Verification items for the finished model (mm, model axes). Coordinates: 2 decimals unless noted, no trailing zeros. Loops run counter-clockwise (first coordinate to the right, second up) from the corner with the lowest first, then second, coordinate; pieces in that order, holes last. Notation, with made-up numbers: (64, -34) - (118, -34) arc R16 cw to (118, -4) - close; hole circle Ø9 at (-1.75, 58.25). An arc over 180 degrees is marked (long way). One line per item, written item: value. Start each with the question number.
(1) Section check A-A (z = 36). Record the boundary of the cut face in (x, y), plus the area to 3 significant figures.
(2) Section check D-D (z = -22.5). Record the boundary of the cut face in (x, y), plus the area to 3 significant figures.
(3) Section check B-B (x = -16). Record the boundary of the cut face in (y, z).
(4) Gauge pin test, flat ends, axial feed: P1, Ø0.6, axis at x = -8, y = 2.5, coming from the -Z side; P2, Ø5, axis at x = -5, z = -17, coming from the +Y side; P3, Ø1, axis at x = -12, y = 3, coming from the -Z side. Record the tip position at first contact, or that the pin passes through.
(5) Thickness scan on probe 1 along X at (y, z) = (1.2, -36); probe 2 along Z at (x, y) = (-16, 1.4); probe 3 along Z at (x, y) = (7, 3.6). Record the ranges inside material, lowest first. Write a range as [from, to].
(6) Section check C-C (y = 2.8). Record the boundary of the cut face in (x, z), plus the area to 3 significant figures.
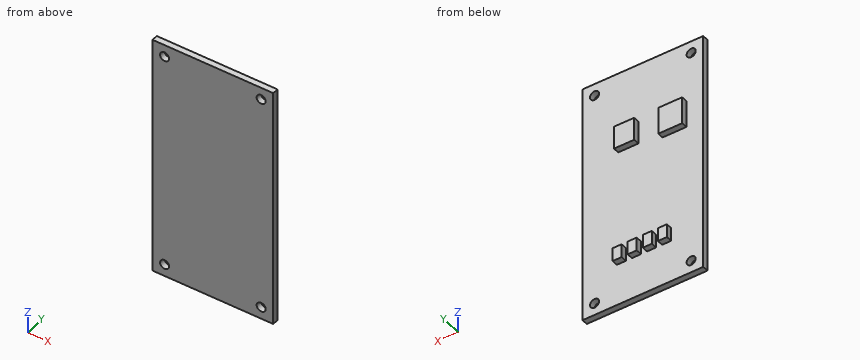
```python
from build123d import *

# Parameters (mm, degrees)
SKETCH_1_W      = 40
SKETCH_1_H      = 80
SKETCH_1_R      = 1.5
EXTRUDE_1_DEPTH = 2
SKETCH_2_W      = 6.701778473
SKETCH_2_H      = 7.607424212
SKETCH_2_W_2    = 7.9099244
SKETCH_2_H_2    = 8.978833102
SKETCH_2_W_3    = 2.99163276
SKETCH_2_H_3    = 4.442525683
EXTRUDE_2_DEPTH = 2


with BuildPart() as part:
    # 草图1 → 凸台-拉伸1 (new body)
    with BuildSketch(Plane(origin=(0, 0, 0), x_dir=(1, 0, 0), z_dir=(0, 1, 0))):
        Rectangle(SKETCH_1_W, SKETCH_1_H)
        with Locations((-16, 36)):
            Circle(SKETCH_1_R, mode=Mode.SUBTRACT)
        with Locations((16, 36)):
            Circle(SKETCH_1_R, mode=Mode.SUBTRACT)
        with Locations((16, -36)):
            Circle(SKETCH_1_R, mode=Mode.SUBTRACT)
        with Locations((-16, -36)):
            Circle(SKETCH_1_R, mode=Mode.SUBTRACT)
    extrude(amount=EXTRUDE_1_DEPTH)

    # 草图2 → 凸台-拉伸2 (add)
    with BuildSketch(Plane(origin=(0, 2, 0), x_dir=(1, 0, 0), z_dir=(0, 1, 0))):
        with Locations((4.815794002, -16.482035575)):
            Rectangle(SKETCH_2_W, SKETCH_2_H)
        with Locations((-10.475305286, -15.552621624)):
            Rectangle(SKETCH_2_W_2, SKETCH_2_H_2)
        with Locations((-7.87829503, 23.838782087)):
            Rectangle(SKETCH_2_W_3, SKETCH_2_H_3)
        with Locations((-2.87829503, 23.838782087)):
            Rectangle(SKETCH_2_W_3, SKETCH_2_H_3)
        with Locations((2.12170497, 23.838782087)):
            Rectangle(SKETCH_2_W_3, SKETCH_2_H_3)
        with Locations((7.12170497, 23.838782087)):
            Rectangle(SKETCH_2_W_3, SKETCH_2_H_3)
    extrude(amount=EXTRUDE_2_DEPTH)


solid = part.part
```
Responses:
1. outline: (-20, 0) - (-17.5, 0) - (-17.5, 2) - (-20, 2) - close; (-14.5, 0) - (14.5, 0) - (14.5, 2) - (-14.5, 2) - close; (17.5, 0) - (20, 0) - (20, 2) - (17.5, 2) - close
1. area: 68.0 mm²
2. outline: (-20, 0) - (20, 0) - (20, 2) - (8.62, 2) - (8.62, 4) - (5.63, 4) - (5.63, 2) - (3.62, 2) - (3.62, 4) - (0.63, 4) - (0.63, 2) - (-1.38, 2) - (-1.38, 4) - (-4.37, 4) - (-4.37, 2) - (-6.38, 2) - (-6.38, 4) - (-9.37, 4) - (-9.37, 2) - (-20, 2) - close
2. area: 104 mm²
3. outline: (0, -40) - (2, -40) - (2, -37.5) - (0, -37.5) - close; (0, -34.5) - (2, -34.5) - (2, 34.5) - (0, 34.5) - close; (0, 37.5) - (2, 37.5) - (2, 40) - (0, 40) - close
4. P1: stops at z = -26.06
4. P2: stops at y = 2
4. P3: stops at z = 11.06
5. probe 1: x = [-20, -17.5], [-14.5, 14.5], [17.5, 20]
5. probe 2: z = [-40, -37.5], [-34.5, 34.5], [37.5, 40]
5. probe 3: z = [-26.06, -21.62], [12.68, 20.29]
6. outline: (-14.43, 11.06) - (-6.52, 11.06) - (-6.52, 20.04) - (-14.43, 20.04) - close; (-9.37, -26.06) - (-6.38, -26.06) - (-6.38, -21.62) - (-9.37, -21.62) - close; (-4.37, -26.06) - (-1.38, -26.06) - (-1.38, -21.62) - (-4.37, -21.62) - close; (0.63, -26.06) - (3.62, -26.06) - (3.62, -21.62) - (0.63, -21.62) - close; (1.46, 12.68) - (8.17, 12.68) - (8.17, 20.29) - (1.46, 20.29) - close; (5.63, -26.06) - (8.62, -26.06) - (8.62, -21.62) - (5.63, -21.62) - close
6. area: 175 mm²
